Input: dimensioned drawing with shaded views. Units: mm. Origin: part minimum x, y, z. A direction names the side the tool comes from. Coordinates: 2 decimals unless noted, no trailing zeros. Loops run counter-clockwise (first coordinate to the right, second up) from the corner with the lowest first, then second, coordinate; pieces in that order, holes last.
Item 1: Section query A-A, the plane y = 11. Return the cut outline in (x, z).
Item 2: Line query: probe 1 along X at (y, z) = (11, 4.25); probe 2 along Y at (x, z) = (16, 4.75) (1 decimal); probe 3 along X at (y, z) = (20, 8.5) (1 decimal). Output: solid intervals per line, ascending.
Item 3: Section query C-C, the plane x = 22.5. Return the cut outline in (y, z) (1 decimal), then the cut area to 3 significant figures.
Item 4: Reachability of the marked faces 1, 2 and 3 from +Z, -Z, +X, -X, +Y, -Y: full face, straight path, thin tool, end or side. Return the list, or none.
Item 5: Pin query (flat end, axial travel): pin 1 Ø3 at (y, z) = (11, 4.5) entering from +X; pin 2 Ø2 at (x, y) = (19, 26) entering from +Z; pin 3 Ø1.5 at (x, z) = (16, 7) entering from +Y; pin 4 Ø4.5 at (y, z) = (32.5, 5) entering from -X (1 decimal). Return the tip coordinate at first contact, or that it passes through.
Item 6: Pull-direction query (X, two-part tool) for the marked faces 4, 5 and 6; classes: +X half, -X half, draft (parallel to the pull), parting line (faces both ways), or undercut.
Item 7: Section query D-D, the plane y = 19. Return the cut outline in (x, z).
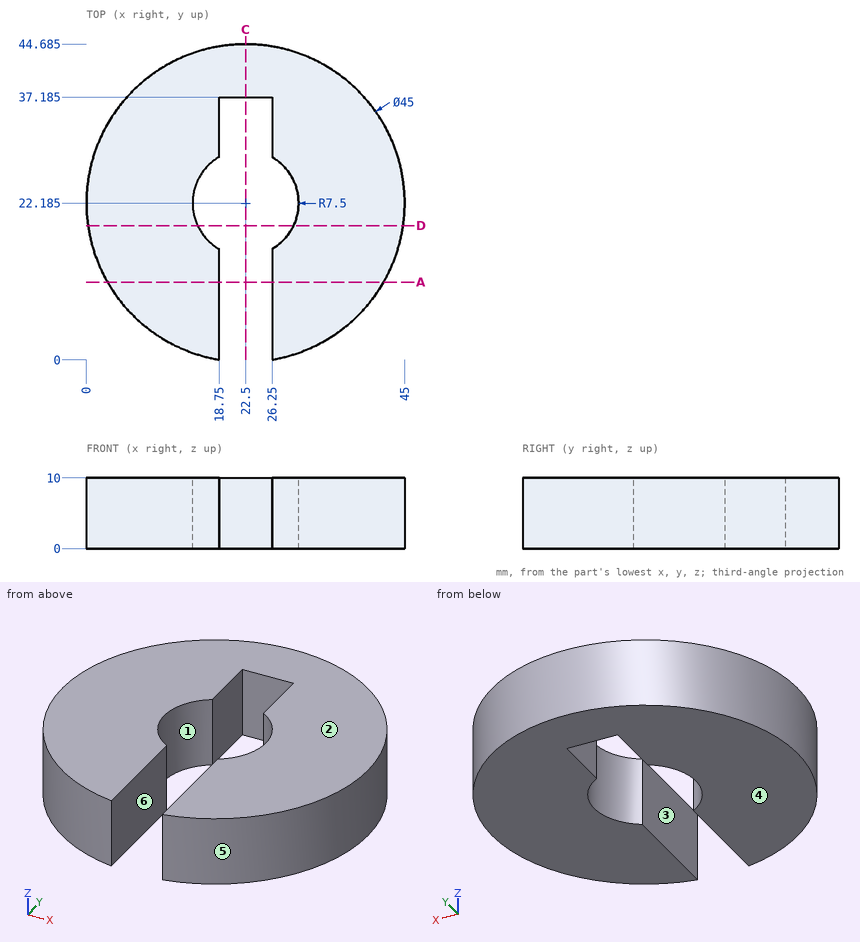
Verdict:
1. outline: (2.98, 0) - (18.75, 0) - (18.75, 10) - (2.98, 10) - close; (26.25, 0) - (42.02, 0) - (42.02, 10) - (26.25, 10) - close
2. probe 1: x = 2.98 to 18.75, 26.25 to 42.02
2. probe 2: y = 0.6 to 18.4, 25.9 to 43.7
2. probe 3: x = 0.1 to 15.3, 29.7 to 44.9
3. outline: (37.2, 0) - (44.7, 0) - (44.7, 10) - (37.2, 10) - close
3. area: 75.0 mm2
4. face 1: +Z, -Z
4. face 2: +Z, +X, -X, +Y, -Y
4. face 3: +Z, -Z, -Y
5. pin 1: stops at x = 42.81
5. pin 2: passes through
5. pin 3: stops at y = 43.94
5. pin 4: stops at x = 1.5
6. face 4: draft
6. face 5: parting line
6. face 6: undercut
7. outline: (0.23, 0) - (15.71, 0) - (15.71, 10) - (0.23, 10) - close; (29.29, 0) - (44.77, 0) - (44.77, 10) - (29.29, 10) - close
